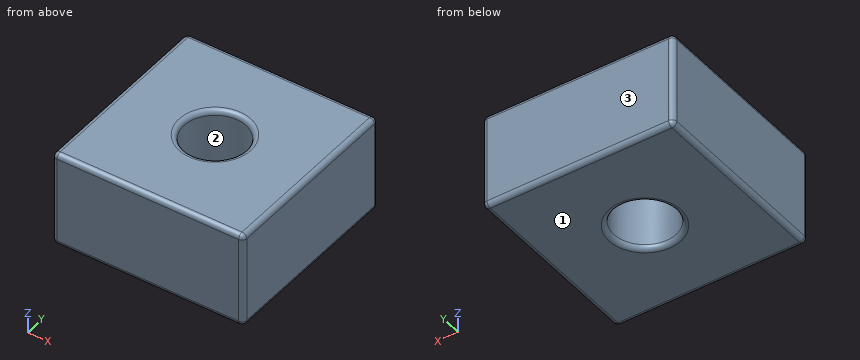
from build123d import *

# Parameters (mm, degrees)
ESQUISSE1_W        = 20
ESQUISSE1_H        = 20
ESQUISSE1_R        = 3.25
BOSS_EXTRU_1_DEPTH = 10
CONG_1_R           = 0.5


with BuildPart() as part:
    # Esquisse1 → Boss.-Extru.1 (new body)
    with BuildSketch(Plane.XY):
        Rectangle(ESQUISSE1_W, ESQUISSE1_H)
        Circle(ESQUISSE1_R, mode=Mode.SUBTRACT)
    extrude(amount=BOSS_EXTRU_1_DEPTH)

    # Congé1
    cong_1_edges = [part.edges().sort_by_distance(p)[0] for p in [
        (-3.25, 0, 0),
        (-3.25, 0, 10),
        (10, 0, 10),
        (0, 10, 10),
        (-10, 0, 10),
        (0, 10, 0),
        (10, 0, 0),
        (0, -10, 0),
        (-10, 0, 0),
        (-10, 10, 5),
        (10, 10, 5),
        (10, -10, 5),
        (-10, -10, 5),
        (0, -10, 10),
    ]]
    fillet(cong_1_edges, radius=CONG_1_R)


solid = part.part
Input: part model. Units: mm. Frame: model coordinates. Face numbers are marked on the shaded views. Round coordinates to 2 decimals unless told otherwise and drop trailing zeros. Order: outer loops, then holes, each group sorted by start corner. A loop starts at its lowest first (then second) coordinate and runs counter-clockwise, first axis right, second up. Notation, with made-up numbers: (-8.75, 82) - (18.25, 82) arc R19 cw to (18.25, 95) - close; hole circle Ø2 at (28.5, 87.5). An arc over 180 degrees is marked (long way). Use a Markdown table: item, result.
1. Section A-A on y = 0. Return the cut outline in (x, z), then the cut area to 3 significant figures.
Evaluation:
| item | result |
|---|---|
| outline | (-10, 0.5) arc R0.5 ccw to (-9.5, 0) - (-3.75, 0) arc R0.5 ccw to (-3.25, 0.5) - (-3.25, 9.5) arc R0.5 ccw to (-3.75, 10) - (-9.5, 10) arc R0.5 ccw to (-10, 9.5) - close; (3.25, 0.5) arc R0.5 ccw to (3.75, 0) - (9.5, 0) arc R0.5 ccw to (10, 0.5) - (10, 9.5) arc R0.5 ccw to (9.5, 10) - (3.75, 10) arc R0.5 ccw to (3.25, 9.5) - close |
| area | 135 mm^2 |
2. Material intervals for probe 1 along Y at (x, z) = (0, 6.5); probe 2 along X at (y, z) = (-1.25, 3.75); probe 3 along Y at (x, z) = (-2.75, 4.25), sorted ascending.
Evaluation:
| item | result |
|---|---|
| probe 1 | -10 to -3.25, 3.25 to 10 |
| probe 2 | -10 to -3, 3 to 10 |
| probe 3 | -10 to -1.73, 1.73 to 10 |
3. Section D-D on z = 9.75. Return the cut outline in (x, y).
Evaluation:
| item | result |
|---|---|
| outline | (-9.93, -9.5) arc R0.43 ccw to (-9.5, -9.93) - (9.5, -9.93) arc R0.43 ccw to (9.93, -9.5) - (9.93, 9.5) arc R0.43 ccw to (9.5, 9.93) - (-9.5, 9.93) arc R0.43 ccw to (-9.93, 9.5) - close; hole circle Ø6.63 at (0, 0) |
4. Mould query, pull axis Y, two halves, no side actions, for the marked faces 1, 2 and 3. Classes: +Y half, -Y half, draft (parallel to the pull), parting line (faces both ways), or undercut.
Evaluation:
| item | result |
|---|---|
| face 1 | draft |
| face 2 | undercut |
| face 3 | +Y half |
5. Section C-C on z = 1.75. Return the cut outline in (x, y), then the cut area to 3 significant figures.
Evaluation:
| item | result |
|---|---|
| outline | (-10, -9.5) arc R0.5 ccw to (-9.5, -10) - (9.5, -10) arc R0.5 ccw to (10, -9.5) - (10, 9.5) arc R0.5 ccw to (9.5, 10) - (-9.5, 10) arc R0.5 ccw to (-10, 9.5) - close; hole circle Ø6.5 at (0, 0) |
| area | 367 mm^2 |
